The model under review builds one solid part; all positions refer to its coordinate system, in mm. A direction names the side the tool comes from. Round coordinates to 2 decimals unless told otherwise and drop trailing zeros.
1) Consider section A-A (y = -9.25). Give the number of separate pieces and of enclosed holes in the cut face, then the cut area to 3 significant figures.
2) To check wall thickness, follow L1, parallel to X at y = -7, z = -17; L2, parallel to X at y = -5.25, z = -33.5; L3, parallel to X at y = -12, z = -51.5. State the ranges of each line that lie inside material, in increasing order.
3) Clearance check with flat-ended pins moving along their axes: P1, Ø6, axis at y = -5, z = -16, coming from the -X side; P2, Ø4, axis at x = -10, y = -16.5, coming from the -Z side; P3, Ø5, axis at y = -9, z = -46, coming from the -X side; P4, Ø5.5, axis at x = -14.03, z = 52.33, coming from the -Y side. State where each tip first meets the part, or that it passes through.
4) Mouldability with a two-part tool opening along X and no side actions: class faces 1 (the face through (-3, -25.4, 2)), 2 (the face through (-0.4, -12.5, 59.6)), 3 (the face through (9.099, -12.522, -70.928)) as pulls with the +X half, pulls with the -X half, needs draft (parallel to the pull), parting line crosses it, or undercut.
5) Machinability: for faces 4 (the face through (-23, -12.7, 14)), 5 (the face through (-13.183, -12.522, -70.423)), which of the approach directions +Z, -Z, +X, -X, +Y, -Y give a long, thin tool a straight path to every point of the face, cutting with its end or side? Answer none if there is none.
from build123d import *

# Parameters (mm, degrees)
F0_R     = 2.9494351417
F0_R_2   = 3.1269179554
F1_DEPTH = 25.4
F2_DEPTH = 12.7


with BuildPart() as f1:
    # F0 (on Front) → F1 (new body)
    with BuildSketch(Plane.XZ):
        with BuildLine():
            add(Edge.make_bspline(
                [(-4.3607349508, 34.3170873821), (-5.8159647731, 34.266180532), (-7.3260798919, 34.6754060156), (-8.8239335735, 35.4499210748)],
                knots=[0, 0, 0, 0, 0.0558604963, 0.0558604963, 0.0558604963, 0.0558604963], degree=3))
            add(Edge.make_bspline(
                [(0, 35.9002791652), (-1.3646498289, 34.9315221296), (-2.8324242194, 34.3705507485), (-4.3607349508, 34.3170873821)],
                knots=[0.9413342177, 0.9413342177, 0.9413342177, 0.9413342177, 1, 1, 1, 1], degree=3))
            add(Edge.make_bspline(
                [(8.1590511892, 61.9637204051), (9.1888372029, 56.929624723), (7.6915449767, 45.4957659335), (2.7445864281, 37.8486452262), (0, 35.9002791652)],
                knots=[0.6905514826, 0.6905514826, 0.6905514826, 0.6905514826, 0.8233454805, 0.9413342177, 0.9413342177, 0.9413342177, 0.9413342177], degree=3))
            add(Edge.make_bspline(
                [(-22.0211678961, 58.0308431791), (-22.1869263998, 61.722066111), (-19.4617275875, 72.4905198421), (2.6471335613, 74.9151403272), (7.5068546983, 65.1519745619), (8.1590511892, 61.9637204051)],
                knots=[0.2961980111, 0.2961980111, 0.2961980111, 0.2961980111, 0.395080951, 0.6064487872, 0.6905514826, 0.6905514826, 0.6905514826, 0.6905514826], degree=3))
            add(Edge.make_bspline(
                [(-22.0211678961, 58.0308431791), (-21.0930203688, 54.6165518536), (-20.1646660473, 51.2021484936), (-19.3839201593, 47.8835665328)],
                knots=[0, 0, 0, 0, 0.1273376133, 0.1273376133, 0.1273376133, 0.1273376133], degree=3))
            add(Edge.make_bspline(
                [(-8.8239335735, 35.4499210748), (-12.3821829949, 37.2898322723), (-16.3569635, 41.7343103663), (-19.07368946, 47.2040259263), (-19.3839201593, 47.8835665328)],
                knots=[0.0558604963, 0.0558604963, 0.0558604963, 0.0558604963, 0.1885607602, 0.207034532, 0.207034532, 0.207034532, 0.207034532], degree=3))
        make_face()
        with Locations((-14.0301892534, 52.3288138211)):
            Circle(F0_R, mode=Mode.SUBTRACT)
        with Locations((0, 56.499954313)):
            Circle(F0_R_2, mode=Mode.SUBTRACT)
        with BuildLine():
            add(Edge.make_bspline(
                [(0, 35.9002791652), (-1.3646498289, 34.9315221296), (-2.8324242194, 34.3705507485), (-4.3607349508, 34.3170873821)],
                knots=[0.9413342177, 0.9413342177, 0.9413342177, 0.9413342177, 1, 1, 1, 1], degree=3))
            add(Edge.make_bspline(
                [(-4.3607349508, 34.3170873821), (-5.8159647731, 34.266180532), (-7.3260798919, 34.6754060156), (-8.8239335735, 35.4499210748)],
                knots=[0, 0, 0, 0, 0.0558604963, 0.0558604963, 0.0558604963, 0.0558604963], degree=3))
            add(Edge.make_bspline(
                [(-8.8239335735, 35.4499210748), (-8.6194381151, 32.1814535678), (-8.3368843444, 27.3494594149), (-9.9219897476, 26.5952865599), (-10.4278437793, 26.3540036976)],
                knots=[0, 0, 0, 0, 0.6809576007, 1, 1, 1, 1], degree=3))
            add(Edge.make_bspline(
                [(-10.4278437793, 26.3540036976), (-13.5372550637, 27.8193594175), (-16.64666634, 29.2847151335), (-18.5805223781, 26.354003713)],
                knots=[0, 0, 0, 0, 0.2894887536, 0.2894887536, 0.2894887536, 0.2894887536], degree=3))
            add(Edge.make_bspline(
                [(-18.5805223882, 26.3540036976), (-18.8474893981, 25.6657310236), (-19.1628757455, 25.0088850241), (-19.5109327232, 24.378981395)],
                knots=[0.4444669687, 0.4444669687, 0.4444669687, 0.4444669687, 0.4834838181, 0.4834838181, 0.4834838181, 0.4834838181], degree=3))
            add(Edge.make_bspline(
                [(-19.5109327232, 24.378981395), (-21.0643674832, 19.9531113363), (-21.5262468174, 11.8158457348), (-21.5533071763, 4.5179931389)],
                knots=[0.3413897295, 0.3413897295, 0.3413897295, 0.3413897295, 0.6348121446, 0.6348121446, 0.6348121446, 0.6348121446], degree=3))
            add(Edge.make_bspline(
                [(-21.5533071763, 4.5179931389), (-21.577792476, -2.0853970393), (-21.1218013847, -10.2228609905), (-20.9127527805, -10.6817670726), (-20.8556875587, -10.8070373535)],
                knots=[0.6348121446, 0.6348121446, 0.6348121446, 0.6348121446, 0.9003125323, 1, 1, 1, 1], degree=3))
            Line((-20.8556875587, -10.8070373535), (-15.0507342077, -10.9744156837))
            Line((-15.0507342077, -10.9744156837), (-11.9681432843, -11.0632982105))
            add(Edge.make_bspline(
                [(-11.9681432843, -11.0632982105), (-11.7523383257, -12.3312092814), (-11.4293724426, -12.803583638), (-10.0912256166, -13.2083445787)],
                knots=[0.2841176244, 0.2841176244, 0.2841176244, 0.2841176244, 0.3781726374, 0.3781726374, 0.3781726374, 0.3781726374], degree=3))
            add(Edge.make_bspline(
                [(-10.0912256166, -13.2083445787), (-6.999042893, -14.1436640549), (1.5139752093, -14.7179432662), (5.1191220991, -13.7446066365)],
                knots=[0.3781726374, 0.3781726374, 0.3781726374, 0.3781726374, 0.5955144721, 0.5955144721, 0.5955144721, 0.5955144721], degree=3))
            add(Edge.make_bspline(
                [(5.1191220991, -13.7446066365), (7.0668957023, -13.2187364147), (7.5820718333, -12.2411203248), (7.8735407442, -10.2589046583)],
                knots=[0.5955144721, 0.5955144721, 0.5955144721, 0.5955144721, 0.7129390047, 0.7129390047, 0.7129390047, 0.7129390047], degree=3))
            Line((7.8735407442, -10.2589046583), (10.0993986167, -10.4179034599))
            Line((10.0993986167, -10.4179034599), (15.5469663441, -10.8070373535))
            add(Edge.make_bspline(
                [(14.2226914281, 18.9650026151), (15.3554039912, 11.4628427606), (15.4511851676, 0.3279027036), (15.5469663441, -10.8070373535)],
                knots=[0.5401467708, 0.5401467708, 0.5401467708, 0.5401467708, 1, 1, 1, 1], degree=3))
            add(Edge.make_bspline(
                [(5.1191220991, 27.4915862828), (7.3468122477, 28.2109019634), (11.5830450619, 29.5787711404), (13.5918597378, 23.1431148181), (14.2226914281, 18.9650026151)],
                knots=[0, 0, 0, 0, 0.2840447381, 0.5401467708, 0.5401467708, 0.5401467708, 0.5401467708], degree=3))
            add(Edge.make_bspline(
                [(0, 35.9002791652), (0.6659120514, 32.1806234635), (1.6838923464, 26.494382766), (4.2363538824, 27.2353298943), (5.1191220991, 27.4915862828)],
                knots=[0, 0, 0, 0, 0.6541502372, 1, 1, 1, 1], degree=3))
        make_face()
        with BuildLine():
            add(Edge.make_bspline(
                [(5.1191220991, -13.7446066365), (5.3204684593, -26.4078442093), (5.6806533545, -49.0608829649), (12.9222659431, -63.3019604329), (16.1157567054, -69.582156837)],
                knots=[0, 0, 0, 0, 0.5590083392, 1, 1, 1, 1], degree=3))
            add(Edge.make_bspline(
                [(-10.0912256166, -13.2083445787), (-6.999042893, -14.1436640549), (1.5139752093, -14.7179432662), (5.1191220991, -13.7446066365)],
                knots=[0.3781726374, 0.3781726374, 0.3781726374, 0.3781726374, 0.5955144721, 0.5955144721, 0.5955144721, 0.5955144721], degree=3))
            add(Edge.make_bspline(
                [(-10.0912256166, -13.2083445787), (-10.0911388765, -26.0813857287), (-10.0909843429, -49.0156260347), (-17.1778871585, -63.310867055), (-20.2868953347, -69.582156837)],
                knots=[0, 0, 0, 0, 0.5613022702, 1, 1, 1, 1], degree=3))
            Line((-20.2868953347, -69.582156837), (-5.8775120415, -71.2885335088))
            add(Edge.make_bspline(
                [(-5.8775120415, -71.2885335088), (-6.2564772228, -69.1830736559), (-7.386907722, -62.90261268), (-3.6582190501, 8.5281088891), (3.2850759179, -63.0431020915), (2.5337375888, -69.8826869928), (2.2751661018, -72.2365155816)],
                knots=[0, 0, 0, 0, 0.1662763633, 0.4959924596, 0.8265468775, 1, 1, 1, 1], degree=3))
            Line((2.2751661018, -72.2365155816), (16.1157567054, -69.582156837))
        make_face()
        with BuildLine():
            add(Edge.make_bspline(
                [(15.5469663441, -10.8070373535), (15.1276841103, -14.9343334931), (14.2669666052, -23.4069940283), (11.5160993619, -14.8561836208), (10.0993986167, -10.4179034599)],
                knots=[0, 0, 0, 0, 0.4841661128, 0.993913443, 0.993913443, 0.993913443, 0.993913443], degree=3))
            Line((15.5469663441, -10.8070373535), (10.0993986167, -10.4179034599))
        make_face()
        with BuildLine():
            Line((-15.0507342077, -10.9744156837), (-20.8556875587, -10.8070373535))
            add(Edge.make_bspline(
                [(-20.8556875587, -10.8070373535), (-20.4670630449, -14.3410148632), (-19.6726079619, -21.5654340555), (-16.6193671781, -14.5925942328), (-15.0507342077, -10.9744156837)],
                knots=[0, 0, 0, 0, 0.4853486561, 0.9921857557, 0.9921857557, 0.9921857557, 0.9921857557], degree=3))
        make_face()
    extrude(amount=F1_DEPTH)

    # F0 (on Front) → F2 (join)
    with BuildSketch(Plane.XZ):
        with BuildLine():
            add(Edge.make_bspline(
                [(-8.8239335735, 35.4499210748), (-8.6194381151, 32.1814535678), (-8.3368843444, 27.3494594149), (-9.9219897476, 26.5952865599), (-10.4278437793, 26.3540036976)],
                knots=[0, 0, 0, 0, 0.6809576007, 1, 1, 1, 1], degree=3))
            add(Edge.make_bspline(
                [(-8.8239335735, 35.4499210748), (-12.3821829949, 37.2898322723), (-16.3569635, 41.7343103663), (-19.07368946, 47.2040259263), (-19.3839201593, 47.8835665328)],
                knots=[0.0558604963, 0.0558604963, 0.0558604963, 0.0558604963, 0.1885607602, 0.207034532, 0.207034532, 0.207034532, 0.207034532], degree=3))
            add(Edge.make_bspline(
                [(-19.3839201593, 47.8835665328), (-17.4395030004, 39.6187676959), (-16.410611773, 31.9482911058), (-18.5805223882, 26.3540036976)],
                knots=[0.1273376133, 0.1273376133, 0.1273376133, 0.1273376133, 0.4444669687, 0.4444669687, 0.4444669687, 0.4444669687], degree=3))
            add(Edge.make_bspline(
                [(-10.4278437793, 26.3540036976), (-13.5372550637, 27.8193594175), (-16.64666634, 29.2847151335), (-18.5805223781, 26.354003713)],
                knots=[0, 0, 0, 0, 0.2894887536, 0.2894887536, 0.2894887536, 0.2894887536], degree=3))
        make_face()
        with BuildLine():
            add(Edge.make_bspline(
                [(-19.5109327232, 24.378981395), (-21.0643674832, 19.9531113363), (-21.5262468174, 11.8158457348), (-21.5533071763, 4.5179931389)],
                knots=[0.3413897295, 0.3413897295, 0.3413897295, 0.3413897295, 0.6348121446, 0.6348121446, 0.6348121446, 0.6348121446], degree=3))
            add(Edge.make_bspline(
                [(-19.5109327232, 24.378981395), (-21.8348555242, 20.1732119385), (-29.3302897757, 14.2158038787), (-24.1232589853, 7.7328778416), (-21.5533071763, 4.5179931389)],
                knots=[0.4834838181, 0.4834838181, 0.4834838181, 0.4834838181, 0.7439933089, 1, 1, 1, 1], degree=3))
        make_face()
        with BuildLine():
            add(Edge.make_bspline(
                [(8.1590511892, 61.9637204051), (9.1888372029, 56.929624723), (7.6915449767, 45.4957659335), (2.7445864281, 37.8486452262), (0, 35.9002791652)],
                knots=[0.6905514826, 0.6905514826, 0.6905514826, 0.6905514826, 0.8233454805, 0.9413342177, 0.9413342177, 0.9413342177, 0.9413342177], degree=3))
            add(Edge.make_bspline(
                [(0, 35.9002791652), (0.6659120514, 32.1806234635), (1.6838923464, 26.494382766), (4.2363538824, 27.2353298943), (5.1191220991, 27.4915862828)],
                knots=[0, 0, 0, 0, 0.6541502372, 1, 1, 1, 1], degree=3))
            add(Edge.make_bspline(
                [(5.1191220991, 27.4915862828), (7.3468122477, 28.2109019634), (11.5830450619, 29.5787711404), (13.5918597378, 23.1431148181), (14.2226914281, 18.9650026151)],
                knots=[0, 0, 0, 0, 0.2840447381, 0.5401467708, 0.5401467708, 0.5401467708, 0.5401467708], degree=3))
            add(Edge.make_bspline(
                [(8.1590511892, 61.9637204051), (12.6372937315, 53.5646840832), (20.9003420601, 38.0594699763), (16.3294038546, 24.9669144954), (14.2226914281, 18.9650026151)],
                knots=[0, 0, 0, 0, 0.5415898832, 1, 1, 1, 1], degree=3))
        make_face()
    extrude(amount=F2_DEPTH)


solid = f1.part
Answer below:
1. separate pieces: 1
1. enclosed holes: 2
1. area: 3,760 mm2
2. L1: x = -19.88 to -17.97, -10.09 to 5.17, 12.37 to 14.77
2. L2: x = -10.44 to -5.45, 0.02 to 5.76
2. L3: x = -12.9 to -6.45, 1.84 to 8.49
3. P1: stops at x = -20.61
3. P2: stops at z = -71.04
3. P3: stops at x = -12.19
3. P4: passes through
4. face 1: needs draft
4. face 2: undercut
4. face 3: pulls with the +X half
5. face 4: -X, -Y
5. face 5: -Z, -X, +Y, -Y
